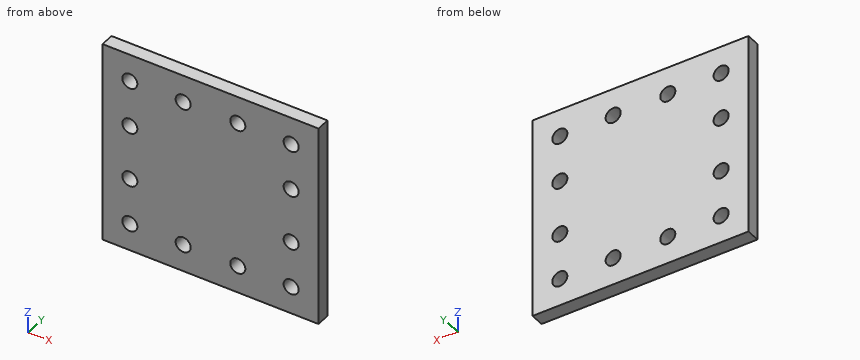
from build123d import *

# Parameters (mm, degrees)
SKETCH1_W           = 100.4
SKETCH1_H           = 93.9
BOSS_EXTRUDE1_DEPTH = 6.35
SKETCH2_R           = 3.5
CUT_EXTRUDE1_DEPTH  = 6.35
SKETCH4_R           = 3.5
CUT_EXTRUDE2_DEPTH  = 6.35


with BuildPart() as part:
    # Sketch1 → Boss-Extrude1 (new body)
    with BuildSketch(Plane(origin=(0, 0, 0), x_dir=(1, 0, 0), z_dir=(0, 1, 0))):
        with Locations((50.2, 46.95)):
            Rectangle(SKETCH1_W, SKETCH1_H)
    extrude(amount=BOSS_EXTRUDE1_DEPTH)

    # Sketch2 → Cut-Extrude1 (cut)
    with BuildSketch(Plane(origin=(0, 6.35, 0), x_dir=(1, 0, 0), z_dir=(0, 1, 0))):
        with Locations(Location((12.7, 81.2, 0), (0, 0, 270))):
            Circle(SKETCH2_R)
        with Locations(Location((12.7, 12.7, 0), (0, 0, 90))):
            Circle(SKETCH2_R)
        with Locations(Location((87.7, 12.7, 0), (0, 0, 270))):
            Circle(SKETCH2_R)
        with Locations(Location((87.7, 81.2, 0), (0, 0, 90))):
            Circle(SKETCH2_R)
    extrude(amount=-CUT_EXTRUDE1_DEPTH, mode=Mode.SUBTRACT)

    # Sketch4 → Cut-Extrude2 (cut)
    with BuildSketch(Plane(origin=(0, 6.35, 0), x_dir=(1, 0, 0), z_dir=(0, 1, 0))):
        with Locations(Location((12.7, 59.65, 0), (0, 0, 270))):
            Circle(SKETCH4_R)
        with Locations(Location((12.7, 34.25, 0), (0, 0, 90))):
            Circle(SKETCH4_R)
        with Locations(Location((87.7, 34.25, 0), (0, 0, 270))):
            Circle(SKETCH4_R)
        with Locations(Location((87.7, 59.65, 0), (0, 0, 90))):
            Circle(SKETCH4_R)
        with Locations(Location((37.5, 81.2, 0), (0, 0, 270))):
            Circle(SKETCH4_R)
        with Locations(Location((62.9, 81.2, 0), (0, 0, 90))):
            Circle(SKETCH4_R)
        with Locations(Location((62.9, 12.7, 0), (0, 0, 270))):
            Circle(SKETCH4_R)
        with Locations(Location((37.5, 12.7, 0), (0, 0, 90))):
            Circle(SKETCH4_R)
    extrude(amount=-CUT_EXTRUDE2_DEPTH, mode=Mode.SUBTRACT)


solid = part.part
Model file for the job. Use its own axes, mm. Give positions to 0.01 mm unless a question says otherwise; leave off trailing zeros. Write each loop counter-clockwise with the first axis right and the second up, starting at its lowest first coordinate (ties: lowest second). Pieces come first, ordered by that corner, then holes. Notation, with made-up numbers: (58, -0.5) -> (91, -0.5) arc R20 cw to (91, 20.5) -> close; hole circle Ø6 at (12.5, 69.25). An arc over 180 degrees is marked (long way). Write item = value, one per line.
(1) Flat gauge pins, fed straight in: P1, Ø6, axis at x = 52, z = -43, coming from the -Y side; P2, Ø4, axis at x = 62.9, z = -81.2, coming from the -Y side. Where does each tip first touch, or does it go through?
Determined:
P1 = 0
P2 = through
(2) Slice it at B-B, the plane z = -81.2. Give the cut face in (x, y), then the cut area to 3 significant figures.
Determined:
outline = (0, 0) -> (9.2, 0) -> (9.2, 6.35) -> (0, 6.35) -> close; (16.2, 0) -> (34, 0) -> (34, 6.35) -> (16.2, 6.35) -> close; (41, 0) -> (59.4, 0) -> (59.4, 6.35) -> (41, 6.35) -> close; (66.4, 0) -> (84.2, 0) -> (84.2, 6.35) -> (66.4, 6.35) -> close; (91.2, 0) -> (100.4, 0) -> (100.4, 6.35) -> (91.2, 6.35) -> close
area = 460 mm2
(3) Slice it at A-A, the plane z = -34.25. Give the cut face in (x, y).
Determined:
outline = (0, 0) -> (9.2, 0) -> (9.2, 6.35) -> (0, 6.35) -> close; (16.2, 0) -> (84.2, 0) -> (84.2, 6.35) -> (16.2, 6.35) -> close; (91.2, 0) -> (100.4, 0) -> (100.4, 6.35) -> (91.2, 6.35) -> close
(4) Slice it at C-C, the plane y = 4. Give the number of separate pieces and of enclosed holes in the cut face, then the cut area to 3 significant figures.
Determined:
separate_pieces = 1
enclosed_holes = 12
area = 8,970 mm2
(5) Slice it at D-D, the plane x = 62.9. Give the cut face in (y, z), then the cut area to 3 significant figures.
Determined:
outline = (0, -93.9) -> (6.35, -93.9) -> (6.35, -84.7) -> (0, -84.7) -> close; (0, -77.7) -> (6.35, -77.7) -> (6.35, -16.2) -> (0, -16.2) -> close; (0, -9.2) -> (6.35, -9.2) -> (6.35, 0) -> (0, 0) -> close
area = 507 mm2
(6) Probe line 1 along X through (y, z) = (5.25, -81.2); line 2 along X through (y, z) = (3, -59.65); line 3 along X through (y, z) = (3.5, -37). List the from-to ranges inside material, lowest first.
Determined:
line_1 = 0 to 9.2, 16.2 to 34, 41 to 59.4, 66.4 to 84.2, 91.2 to 100.4
line_2 = 0 to 9.2, 16.2 to 84.2, 91.2 to 100.4
line_3 = 0 to 10.53, 14.87 to 85.53, 89.87 to 100.4
